CAD build for the part. Positions are in the model's coordinates, mm. Face numbers are marked on the shaded views. A direction names the side the tool comes from. Coordinates: 2 decimals unless noted, no trailing zeros. Loops run counter-clockwise (first coordinate to the right, second up) from the corner with the lowest first, then second, coordinate; pieces in that order, holes last. Notation, with made-up numbers: (41.25, 0) -> (49.25, 0) arc R34 cw to (49.25, 31) -> close; hole circle Ø4 at (4, -39). An arc over 180 degrees is marked (long way). Return JSON: item names as keys, results as strings. Group by question number.
(1) Saw through at A-A on y = 16. Write the cut outline in (x, z), then the cut area to 3 significant figures.
(2) Mould opens along Y. For the marked faces 1, 2 and 3 say: pulls with the +Y half, pulls with the -Y half, needs draft (parallel to the pull), parting line crosses it, or undercut.
(3) Saw through at C-C on x = 4.2. Give the number of separate pieces and of enclosed holes in the cut face, then the cut area to 3 significant figures.
(4) Saw through at D-D on y = 9.25. Write the cut outline in (x, z), then the cut area to 3 significant figures.
(5) Saw through at B-B on z = -2.25. Write the cut outline in (x, y).
(6) Probe L1, parallel to Z at x = 4.2, y = 10.5; L2, parallel to X at y = 10.75, z = -17.7; L3, parallel to Z at x = 5.25, y = 8.5. List the from-to ranges inside material, lowest first.
(7) Flat gauge pins, fed straight in: pin 1 Ø3 at (x, z) = (4, -17.5) entering from +Y; pin 2 Ø4 at (x, y) = (4.5, 1.5) entering from -Z; pin 3 Ø2 at (x, y) = (2, 15) entering from +Z. Where does each tip first touch, or does it go through?
(8) Tool access for the marked faces 4, 5 and 6: list every direction of +Z, -Z, +X, -X, +Y, -Y with a clear straight run to the whole face (end or side of a thin tool).
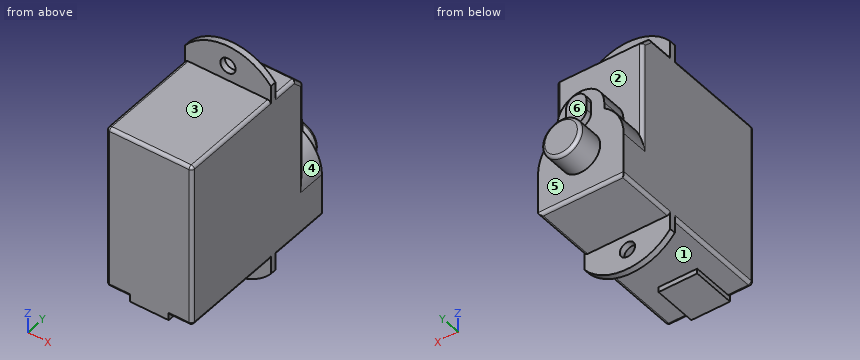
```python
from build123d import *

# Parameters (mm, degrees)
SKETCH_1_W      = 8.4
SKETCH_1_H      = 16.2
EXTRUDE_1_DEPTH = 14.5
SKETCH_3_R      = 0.75
EXTRUDE_2_DEPTH = 0.6
EXTRUDE_3_DEPTH = 2.5
SKETCH_5_R      = 1.9
EXTRUDE_4_DEPTH = 2.6
EXTRUDE_5_DEPTH = 0.6
EXTRUDE_6_DEPTH = 0.5
CHAMFER_1_SIZE  = 1
FILLET_1_R      = 0.3


with BuildPart() as part:
    # 草图1 → 凸台-拉伸1 (new body)
    with BuildSketch(Plane(origin=(0, 0, 0), x_dir=(1, 0, 0), z_dir=(0, 1, 0))):
        with Locations((4.2, 8.1)):
            Rectangle(SKETCH_1_W, SKETCH_1_H)
    extrude(amount=EXTRUDE_1_DEPTH)

    # 草图3 → 凸台-拉伸2 (add)
    with BuildSketch(Plane(origin=(0, 10.3, 0), x_dir=(-1, 0, 0), z_dir=(0, -1, 0))):
        with BuildLine():
            Line((0, 16.2), (0, 17.7))
            ThreePointArc((0, 17.7), (-4.2, 19.7), (-8.4, 17.7))
            Line((-8.4, 17.7), (-8.4, 16.2))
            Line((-8.4, 16.2), (0, 16.2))
        make_face()
        with Locations((-4.2, 17.7)):
            Circle(SKETCH_3_R, mode=Mode.SUBTRACT)
        with BuildLine():
            Line((-8.4, 0), (0, 0))
            Line((0, 0), (0, -1.5))
            ThreePointArc((0, -1.5), (-4.2, -3.5), (-8.4, -1.5))
            Line((-8.4, -1.5), (-8.4, 0))
        make_face()
        with Locations((-4.2, -1.5)):
            Circle(SKETCH_3_R, mode=Mode.SUBTRACT)
    extrude(amount=-EXTRUDE_2_DEPTH)

    # 草图4 → 凸台-拉伸3 (add)
    with BuildSketch(Plane(origin=(0, 14.5, 0), x_dir=(1, 0, 0), z_dir=(0, 1, 0))):
        with BuildLine():
            Line((8.4, 12), (8.4, 16.2))
            Line((8.4, 16.2), (0, 16.2))
            Line((0, 16.2), (0, 12))
            ThreePointArc((0, 12), (0.50540936, 10.002501564), (1.9, 8.485743322))
            Line((1.9, 8.485743322), (1.9, 7.9))
            ThreePointArc((1.9, 7.9), (4.2, 5.6), (6.5, 7.9))
            Line((6.5, 7.9), (6.5, 8.485743322))
            ThreePointArc((6.5, 8.485743322), (7.89459064, 10.002501564), (8.4, 12))
        make_face()
    extrude(amount=EXTRUDE_3_DEPTH)

    # 草图5 → 凸台-拉伸4 (add)
    with BuildSketch(Plane(origin=(0, 17, 0), x_dir=(1, 0, 0), z_dir=(0, 1, 0))):
        with Locations((4.2, 12)):
            Circle(SKETCH_5_R)
    extrude(amount=EXTRUDE_4_DEPTH)

    # 草图6 → 凸台-拉伸5 (add)
    with BuildSketch(Plane(origin=(0, 17, 0), x_dir=(1, 0, 0), z_dir=(0, 1, 0))):
        with BuildLine():
            Line((5.2, 8.35), (5.2, 7.35))
            ThreePointArc((5.2, 7.35), (4.2, 6.35), (3.2, 7.35))
            Line((3.2, 7.35), (3.2, 8.35))
            ThreePointArc((3.2, 8.35), (4.2, 9.35), (5.2, 8.35))
        make_face()
    extrude(amount=EXTRUDE_5_DEPTH)

    # 草图7 → 凸台-拉伸6 (add)
    with BuildSketch(Plane(origin=(0, 0, -16.2), x_dir=(-1, 0, 0), z_dir=(0, 0, -1))):
        Polygon((-4.2, 4.3), (-6.1, 4.3), (-6.1, 0), (-2.3, 0), (-2.3, 4.3), align=None)
    extrude(amount=EXTRUDE_6_DEPTH)

    # 倒角1
    chamfer_1_edges = [part.edges().sort_by_distance(p)[0] for p in [
        (4.2, 14.5, 0),
    ]]
    chamfer(chamfer_1_edges, length=CHAMFER_1_SIZE)

    # 圆角1
    fillet_1_edges = [part.edges().sort_by_distance(p)[0] for p in [
        (1.15, 0, -16.2),
        (8.4, 14.5, -6.5),
        (8.4, 12.2, 0),
        (8.4, 14, -0.5),
        (0, 12.2, 0),
        (0, 14, -0.5),
        (0, 5.15, -16.2),
        (8.4, 5.15, -16.2),
        (8.4, 5.15, 0),
        (0, 5.15, 0),
        (0, 14.5, -6.5),
        (0, 0, -8.1),
        (4.2, 17, -16.2),
        (7.25, 0, -16.2),
        (8.4, 0, -8.1),
        (4.2, 0, 0),
        (2.3, 19.6, -12),
        (0, 13.95, -16.2),
        (8.4, 13.95, -16.2),
    ]]
    fillet(fillet_1_edges, radius=FILLET_1_R)


solid = part.part
```
Geometry results:
{
 "1": {"outline": "(0, -15.9) arc R0.3 ccw to (0.3, -16.2) -> (8.1, -16.2) arc R0.3 ccw to (8.4, -15.9) -> (8.4, -12) arc R4.2 ccw to (6.5, -8.49) -> (6.5, -7.9) arc R2.3 ccw to (1.9, -7.9) -> (1.9, -8.49) arc R4.2 ccw to (0, -12) -> close", "area": "71.8 mm²"},
 "2": {"face 1": "undercut", "face 2": "pulls with the +Y half", "face 3": "needs draft"},
 "3": {"separate pieces": "3", "enclosed holes": "0", "area": "277 mm²"},
 "4": {"outline": "(0, -15.9) arc R0.3 ccw to (0.3, -16.2) -> (8.1, -16.2) arc R0.3 ccw to (8.4, -15.9) -> (8.4, -0.3) arc R0.3 ccw to (8.1, 0) -> (0.3, 0) arc R0.3 ccw to (0, -0.3) -> close", "area": "136 mm²"},
 "5": {"outline": "(0, 0.3) arc R0.3 ccw to (0.3, 0) -> (8.1, 0) arc R0.3 ccw to (8.4, 0.3) -> (8.4, 14.2) arc R0.3 ccw to (8.1, 14.5) -> (0.3, 14.5) arc R0.3 ccw to (0, 14.2) -> close"},
 "6": {"L1": "-19.7 to -18.45, -16.95 to 0.75, 2.25 to 3.5", "L2": "0 to 3.45, 4.95 to 8.4", "L3": "-16.2 to 0"},
 "7": {"pin 1": "y = 16.98", "pin 2": "z = -16.7", "pin 3": "z = -0.5"},
 "8": {"face 4": "+Z, +X, +Y", "face 5": "+Y", "face 6": "+Z, +X, -X, +Y"}
}
